from build123d import *

# Parameters (mm, degrees)
F0_R     = 220
F1_DEPTH = 8
F2_T     = -3
F3_R     = 130
F4_DEPTH = 8.001


with BuildPart() as f1:
    # F0 (on Front) → F1 (new body)
    with BuildSketch(Plane.XZ):
        Circle(F0_R)
    extrude(amount=F1_DEPTH)

    # F2
    f2_openings = [f1.faces().sort_by_distance(p)[0] for p in [
        (0, -8, 0),
    ]]
    offset(amount=F2_T, openings=f2_openings)

    # F3 (on face) → F4 (cut, through all)
    with BuildSketch(Plane.XZ.offset(8)):
        Circle(F3_R)
    extrude(amount=-F4_DEPTH, mode=Mode.SUBTRACT)


solid = f1.part
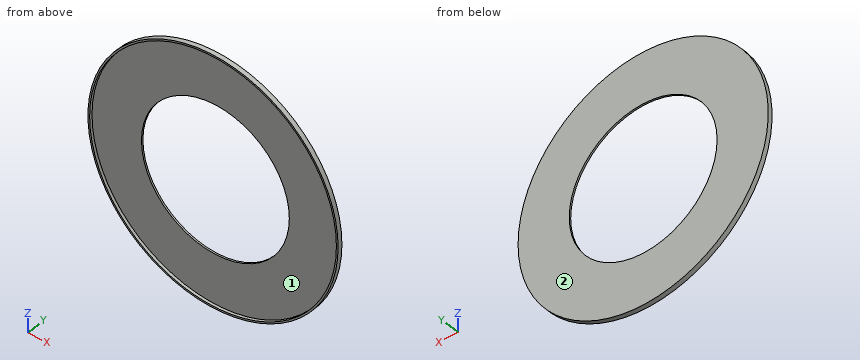
Here's how the part is built. I have some questions about the finished solid (model axes, mm). Face numbers are marked on the shaded views. Coordinates: 2 decimals unless noted, no trailing zeros. Write each loop counter-clockwise with the first axis right and the second up, starting at its lowest first coordinate (ties: lowest second). Pieces come first, ordered by that corner, then holes. Notation, with made-up numbers: (54.5, -23) - (107.5, -23) arc R28 cw to (107.5, 5) - close; hole circle Ø4 at (-38, 2). An arc over 180 degrees is marked (long way). Use one line per item in the form item = value.
1) I need wall thicknesses on line 1 (Z direction, x = 0, y = -2.35); line 2 (Z direction, x = 0, y = -4.7); line 3 (Y direction, x = -157, z = -23). Which ranges of each line are inside material? Lowest first, please.
Solved:
line_1 = -220 to -130, 130 to 220
line_2 = -220 to -217, 217 to 220
line_3 = -3 to 0
2) Suppose I cut it at B-B, the plane z = 0. Write out the boundary of the cut face in (x, y), plus the area to 3 significant figures.
Solved:
outline = (-220, -8) - (-217, -8) - (-217, -3) - (-130, -3) - (-130, 0) - (-220, 0) - close; (130, -3) - (217, -3) - (217, -8) - (220, -8) - (220, 0) - (130, 0) - close
area = 570 mm2
3) Suppose I cut it at A-A, the plane x = 0. Write out the boundary of the cut face in (y, z).
Solved:
outline = (-8, -220) - (0, -220) - (0, -130) - (-3, -130) - (-3, -217) - (-8, -217) - close; (-8, 217) - (-3, 217) - (-3, 130) - (0, 130) - (0, 220) - (-8, 220) - close
4) Thinking about a two-plate mould opening in X: for the marked faces 1 and 2, which applies, released by +X, released by -X, zero draft, split by the parting line, or undercut?
Solved:
face_1 = undercut
face_2 = zero draft
5) I'm going to push flat-ended pins straight in: P1, Ø1, axis at y = -6.5, z = -49, coming from the +X side; P2, Ø1.5, axis at x = -100, y = -1, coming from the -Z side; P3, Ø4, axis at x = 136.5, y = -3, coming from the -Z side. Where does each tip first touch, or does it pass through?
Solved:
P1 = 214.59
P2 = -196.34
P3 = -174.1
6) Suppose I cut it at C-C, the plane y = -6.75. Write out the boundary of the cut face in (x, z).
Solved:
outline = circle Ø440 at (0, 0); hole circle Ø434 at (0, 0)
7) Suppose I cut it at D-D, the plane x = 193. Write out the boundary of the cut face in (y, z), plus the area to 3 significant figures.
Solved:
outline = (-8, -105.6) - (0, -105.6) - (0, 105.6) - (-8, 105.6) - (-8, 99.2) - (-3, 99.2) - (-3, -99.2) - (-8, -99.2) - close
area = 698 mm2
